Build history of the part. All positions in model axes, mm. A direction names the side the tool comes from. Give positions to 0.01 mm unless a question says otherwise; leave off trailing zeros. Order: outer loops, then holes, each group sorted by start corner. A loop starts at its lowest first (then second) coordinate and runs counter-clockwise, first axis right, second up. Notation, with made-up numbers: M 11,46.25 L 36,46.25 A26 cw 36,76.25 Z; hole C -2,-32 d3. An arc over 180 degrees is marked long. One line per item, written item: value. Start each with the question number.
from build123d import *

# Parameters (mm, degrees)
SKETCH2_W           = 100
SKETCH2_H           = 100
BOSS_EXTRUDE1_DEPTH = 20
SKETCH3_W           = 100
SKETCH3_H           = 20
CUT_EXTRUDE1_DEPTH  = 12
SKETCH5_R           = 12.5
CUT_EXTRUDE2_DEPTH  = 6
SKETCH6_R           = 12.5
CUT_EXTRUDE3_DEPTH  = 6
SKETCH7_R           = 12.5
CUT_EXTRUDE4_DEPTH  = 6
SKETCH8_R           = 12.5
CUT_EXTRUDE5_DEPTH  = 6
SKETCH9_R           = 4.5
CUT_EXTRUDE6_DEPTH  = 10
SKETCH10_R          = 4.5
CUT_EXTRUDE7_DEPTH  = 10
SKETCH11_R          = 4.5
CUT_EXTRUDE8_DEPTH  = 10
SKETCH12_R          = 4.5
CUT_EXTRUDE9_DEPTH  = 10
SKETCH13_W          = 10
SKETCH13_H          = 15
CUT_EXTRUDE11_DEPTH = 8
SKETCH15_R          = 2.5
CUT_EXTRUDE13_DEPTH = 16
SKETCH16_W          = 8.1
SKETCH16_H          = 4
CUT_EXTRUDE14_DEPTH = 14
SKETCH17_W          = 10
SKETCH17_H          = 8
CUT_EXTRUDE16_DEPTH = 15
SKETCH19_R          = 2.5
CUT_EXTRUDE17_DEPTH = 16
SKETCH21_W          = 10
SKETCH21_H          = 8
CUT_EXTRUDE19_DEPTH = 15
SKETCH22_W          = 10
SKETCH22_H          = 8
CUT_EXTRUDE20_DEPTH = 15
CUT_EXTRUDE21_START = -16
SKETCH23_R          = 2.5
CUT_EXTRUDE21_DEPTH = 16
CUT_EXTRUDE22_START = -16
SKETCH24_R          = 2.5
CUT_EXTRUDE22_DEPTH = 16
SKETCH25_W          = 8.1
SKETCH25_H          = 4
CUT_EXTRUDE23_DEPTH = 15
SKETCH26_W          = 8.1
SKETCH26_H          = 4
CUT_EXTRUDE24_DEPTH = 15
SKETCH27_W          = 8.1
SKETCH27_H          = 4
CUT_EXTRUDE25_DEPTH = 15
SKETCH28_W          = 100
SKETCH28_H          = 12
CUT_EXTRUDE26_DEPTH = 0.5
SKETCH29_W          = 100
SKETCH29_H          = 12
CUT_EXTRUDE27_DEPTH = 0.5


with BuildPart() as part:
    # Sketch2 → Boss-Extrude1 (new body)
    with BuildSketch(Plane(origin=(0, 0, 0), x_dir=(1, 0, 0), z_dir=(0, 1, 0))):
        with Locations((-37.64268429, -41.588796838)):
            Rectangle(SKETCH2_W, SKETCH2_H)
    extrude(amount=BOSS_EXTRUDE1_DEPTH)

    # Sketch3 → Cut-Extrude1 (cut)
    with BuildSketch(Plane(origin=(0, 20, 0), x_dir=(1, 0, 0), z_dir=(0, 1, 0))):
        with Locations((-37.64268429, -41.588796838)):
            Rectangle(SKETCH3_W, SKETCH3_H)
    extrude(amount=-CUT_EXTRUDE1_DEPTH, mode=Mode.SUBTRACT)

    # Sketch5 → Cut-Extrude2 (cut)
    with BuildSketch(Plane(origin=(0, 20, 0), x_dir=(1, 0, 0), z_dir=(0, 1, 0))):
        with Locations((-7.64268429, -62.088796838)):
            Circle(SKETCH5_R)
    extrude(amount=-CUT_EXTRUDE2_DEPTH, mode=Mode.SUBTRACT)

    # Sketch6 → Cut-Extrude3 (cut)
    with BuildSketch(Plane(origin=(0, 20, 0), x_dir=(1, 0, 0), z_dir=(0, 1, 0))):
        with Locations((-67.64268429, -62.088796838)):
            Circle(SKETCH6_R)
    extrude(amount=-CUT_EXTRUDE3_DEPTH, mode=Mode.SUBTRACT)

    # Sketch7 → Cut-Extrude4 (cut)
    with BuildSketch(Plane(origin=(0, 20, 0), x_dir=(1, 0, 0), z_dir=(0, 1, 0))):
        with Locations((-67.64268429, -21.088796838)):
            Circle(SKETCH7_R)
    extrude(amount=-CUT_EXTRUDE4_DEPTH, mode=Mode.SUBTRACT)

    # Sketch8 → Cut-Extrude5 (cut)
    with BuildSketch(Plane(origin=(0, 20, 0), x_dir=(1, 0, 0), z_dir=(0, 1, 0))):
        with Locations((-7.64268429, -21.088796838)):
            Circle(SKETCH8_R)
    extrude(amount=-CUT_EXTRUDE5_DEPTH, mode=Mode.SUBTRACT)

    # Sketch9 → Cut-Extrude6 (cut)
    with BuildSketch(Plane(origin=(0, 14, 0), x_dir=(1, 0, 0), z_dir=(0, 1, 0))):
        with Locations(Location((-67.64268429, -21.088796838, 0), (0, 0, 270))):
            Circle(SKETCH9_R)
    extrude(amount=-CUT_EXTRUDE6_DEPTH, mode=Mode.SUBTRACT)

    # Sketch10 → Cut-Extrude7 (cut)
    with BuildSketch(Plane(origin=(0, 14, 0), x_dir=(1, 0, 0), z_dir=(0, 1, 0))):
        with Locations(Location((-7.64268429, -21.088796838, 0), (0, 0, 270))):
            Circle(SKETCH10_R)
    extrude(amount=-CUT_EXTRUDE7_DEPTH, mode=Mode.SUBTRACT)

    # Sketch11 → Cut-Extrude8 (cut)
    with BuildSketch(Plane(origin=(0, 14, 0), x_dir=(1, 0, 0), z_dir=(0, 1, 0))):
        with Locations(Location((-7.64268429, -62.088796838, 0), (0, 0, 270))):
            Circle(SKETCH11_R)
    extrude(amount=-CUT_EXTRUDE8_DEPTH, mode=Mode.SUBTRACT)

    # Sketch12 → Cut-Extrude9 (cut)
    with BuildSketch(Plane(origin=(0, 14, 0), x_dir=(1, 0, 0), z_dir=(0, 1, 0))):
        with Locations(Location((-67.64268429, -62.088796838, 0), (0, 0, 270))):
            Circle(SKETCH12_R)
    extrude(amount=-CUT_EXTRUDE9_DEPTH, mode=Mode.SUBTRACT)

    # Sketch13 → Cut-Extrude11 (cut)
    with BuildSketch(Plane.XY.offset(91.588796838)):
        with Locations((-67.64268429, 12.5)):
            Rectangle(SKETCH13_W, SKETCH13_H)
    extrude(amount=-CUT_EXTRUDE11_DEPTH, mode=Mode.SUBTRACT)

    # Sketch15 → Cut-Extrude13 (cut)
    with BuildSketch(Plane.XY.offset(83.588796838)):
        with Locations((-67.64268429, 10)):
            Circle(SKETCH15_R)
    extrude(amount=-CUT_EXTRUDE13_DEPTH, mode=Mode.SUBTRACT)

    # Sketch16 → Cut-Extrude14 (cut)
    with BuildSketch(Plane(origin=(0, 0, 0), x_dir=(-1, 0, 0), z_dir=(0, -1, 0))):
        with Locations((67.64268429, -78.588796838)):
            Rectangle(SKETCH16_W, SKETCH16_H)
    extrude(amount=-CUT_EXTRUDE14_DEPTH, mode=Mode.SUBTRACT)

    # Sketch17 → Cut-Extrude16 (cut)
    with BuildSketch(Plane(origin=(0, 20, 0), x_dir=(1, 0, 0), z_dir=(0, 1, 0))):
        with Locations((-7.64268429, -87.588796838)):
            Rectangle(SKETCH17_W, SKETCH17_H)
    extrude(amount=-CUT_EXTRUDE16_DEPTH, mode=Mode.SUBTRACT)

    # Sketch19 → Cut-Extrude17 (cut)
    with BuildSketch(Plane.XY.offset(83.588796838)):
        with Locations((-7.64268429, 10)):
            Circle(SKETCH19_R)
    extrude(amount=-CUT_EXTRUDE17_DEPTH, mode=Mode.SUBTRACT)

    # Sketch21 → Cut-Extrude19 (cut)
    with BuildSketch(Plane(origin=(0, 20, 0), x_dir=(1, 0, 0), z_dir=(0, 1, 0))):
        with Locations((-67.64268429, 4.411203162)):
            Rectangle(SKETCH21_W, SKETCH21_H)
    extrude(amount=-CUT_EXTRUDE19_DEPTH, mode=Mode.SUBTRACT)

    # Sketch22 → Cut-Extrude20 (cut)
    with BuildSketch(Plane(origin=(0, 20, 0), x_dir=(1, 0, 0), z_dir=(0, 1, 0))):
        with Locations((-7.64268429, 4.411203162)):
            Rectangle(SKETCH22_W, SKETCH22_H)
    extrude(amount=-CUT_EXTRUDE20_DEPTH, mode=Mode.SUBTRACT)

    # Sketch23 → Cut-Extrude21 (cut)
    with BuildSketch(Plane(origin=(0, 0, -0.411203162), x_dir=(-1, 0, 0), z_dir=(0, 0, -1)).offset(CUT_EXTRUDE21_START)):
        with Locations(Location((7.64268429, 10, 0), (0, 0, 180))):
            Circle(SKETCH23_R)
    extrude(amount=CUT_EXTRUDE21_DEPTH, mode=Mode.SUBTRACT)

    # Sketch24 → Cut-Extrude22 (cut)
    with BuildSketch(Plane(origin=(0, 0, -0.411203162), x_dir=(-1, 0, 0), z_dir=(0, 0, -1)).offset(CUT_EXTRUDE22_START)):
        with Locations(Location((67.64268429, 10, 0), (0, 0, 180))):
            Circle(SKETCH24_R)
    extrude(amount=CUT_EXTRUDE22_DEPTH, mode=Mode.SUBTRACT)

    # Sketch25 → Cut-Extrude23 (cut)
    with BuildSketch(Plane(origin=(0, 0, 0), x_dir=(-1, 0, 0), z_dir=(0, -1, 0))):
        with Locations((7.64268429, -78.588796838)):
            Rectangle(SKETCH25_W, SKETCH25_H)
    extrude(amount=-CUT_EXTRUDE23_DEPTH, mode=Mode.SUBTRACT)

    # Sketch26 → Cut-Extrude24 (cut)
    with BuildSketch(Plane(origin=(0, 0, 0), x_dir=(-1, 0, 0), z_dir=(0, -1, 0))):
        with Locations((7.64268429, -4.588796838)):
            Rectangle(SKETCH26_W, SKETCH26_H)
    extrude(amount=-CUT_EXTRUDE24_DEPTH, mode=Mode.SUBTRACT)

    # Sketch27 → Cut-Extrude25 (cut)
    with BuildSketch(Plane(origin=(0, 0, 0), x_dir=(-1, 0, 0), z_dir=(0, -1, 0))):
        with Locations((67.64268429, -4.588796838)):
            Rectangle(SKETCH27_W, SKETCH27_H)
    extrude(amount=-CUT_EXTRUDE25_DEPTH, mode=Mode.SUBTRACT)

    # Sketch28 → Cut-Extrude26 (cut)
    with BuildSketch(Plane.XY.offset(31.588796838)):
        with Locations((-37.64268429, 14)):
            Rectangle(SKETCH28_W, SKETCH28_H)
    extrude(amount=-CUT_EXTRUDE26_DEPTH, mode=Mode.SUBTRACT)

    # Sketch29 → Cut-Extrude27 (cut)
    with BuildSketch(Plane(origin=(0, 0, 51.588796838), x_dir=(-1, 0, 0), z_dir=(0, 0, -1))):
        with Locations((37.64268429, 14)):
            Rectangle(SKETCH29_W, SKETCH29_H)
    extrude(amount=-CUT_EXTRUDE27_DEPTH, mode=Mode.SUBTRACT)


solid = part.part
1) Slice it at B-B (y = 11.25). State how many separate pieces and enclosed holes the cut face has, plus the area to 3 significant figures.
2) Pull direction X, two halves, no side cores. Call faces 1 (the flat face through (-8, 7, 6.589)), 2 (the flat face through (-38, 8, 42)), 3 (the flat face through (-87.643, 7.6, 42.3)): pulls with the +X half, pulls with the -X half, needs draft (parallel to the pull), parting line crosses it, or undercut.
3) Tool access for faces 4 (the cylindrical face through (-9.63, 11.52, 11.15)), 5 (the cylindrical face through (-9.63, 8.48, 82.11)), 6 (the flat face through (-72.643, 13, -4)): list every direction of +Z, -Z, +X, -X, +Y, -Y with a clear straight run to the whole face (end or side of a thin tool).
4) Slice it at A-A (x = -34). List the corners of the cut face in (y, z).
5) Drill centre lines: line 1 (X direction, y = 9.25, z = 85.5); line 2 (Z direction, x = -8, y = 6.5); line 3 (Z direction, x = -23, y = 12.75). Where is each one in solid material? Low to high.
6) Slice it at D-D (z = 49). List the corners of the cut face in (x, y), plus the area to 3 significant figures.
7) Slice it at C-C (z = 10). List the corners of the cut face in (x, y), plus the area to 3 significant figures.
8) Drop flat-ended pins along their axis: P1, Ø6, axis at x = -67.64, y = 10, coming from the -Z side; P2, Ø2.5, axis at x = -67, z = 89, coming from the +Y side; P3, Ø7, axis at x = -67, z = 64.5, coming from the +Y side; P4, Ø1.5, axis at y = 12, z = 50, coming from the +X side. Give the stop position or say it passes through.
Results list:
1. separate pieces: 2
1. enclosed holes: 4
1. area: 6,990 mm²
2. face 1: undercut
2. face 2: needs draft
2. face 3: pulls with the -X half
3. face 4: -Z
3. face 5: +Z
3. face 6: -Z, +Y
4. outline: M 0,-8.41 L 20,-8.41 L 20,31.09 L 8,31.09 L 8,52.09 L 20,52.09 L 20,91.59 L 0,91.59 Z
5. line 1: x = -87.64 to -72.64, -62.64 to -12.64, -2.64 to 12.36
5. line 2: z = -0.41 to 2.59, 6.59 to 16.6, 25.57 to 57.6, 66.57 to 76.59, 80.59 to 83.59
5. line 3: z = -8.41 to 31.09, 52.09 to 91.59
6. outline: M -87.64,0 L 12.36,0 L 12.36,8 L -87.64,8 Z
6. area: 800 mm²
7. outline: M -87.64,0 L 12.36,0 L 12.36,20 L -1.87,20 L -1.87,14 L -13.41,14 L -13.41,20 L -61.87,20 L -61.87,14 L -73.41,14 L -73.41,20 L -87.64,20 Z; hole C -67.64,10 d5; hole C -7.64,10 d5
7. area: 1,820 mm²
8. P1: stops at z = -0.41
8. P2: stops at y = 5
8. P3: stops at y = 14
8. P4: passes through
